Geometry check sheet. Reference: drawing and pictorial views, mm from the part's lowest x, y, z. A direction names the side the tool comes from. Give positions to 0.01 mm unless a question says otherwise; leave off trailing zeros. Order: outer loops, then holes, each group sorted by start corner. A loop starts at its lowest first (then second) coordinate and runs counter-clockwise, first axis right, second up. Notation, with made-up numbers: M 80,2 L 122,2 A29 cw 122,34 Z; hole C 16.25,19 d5. An arc over 180 degrees is marked long. Use CSV: the item, a comma, the result in double quotes. Start each with the question number.
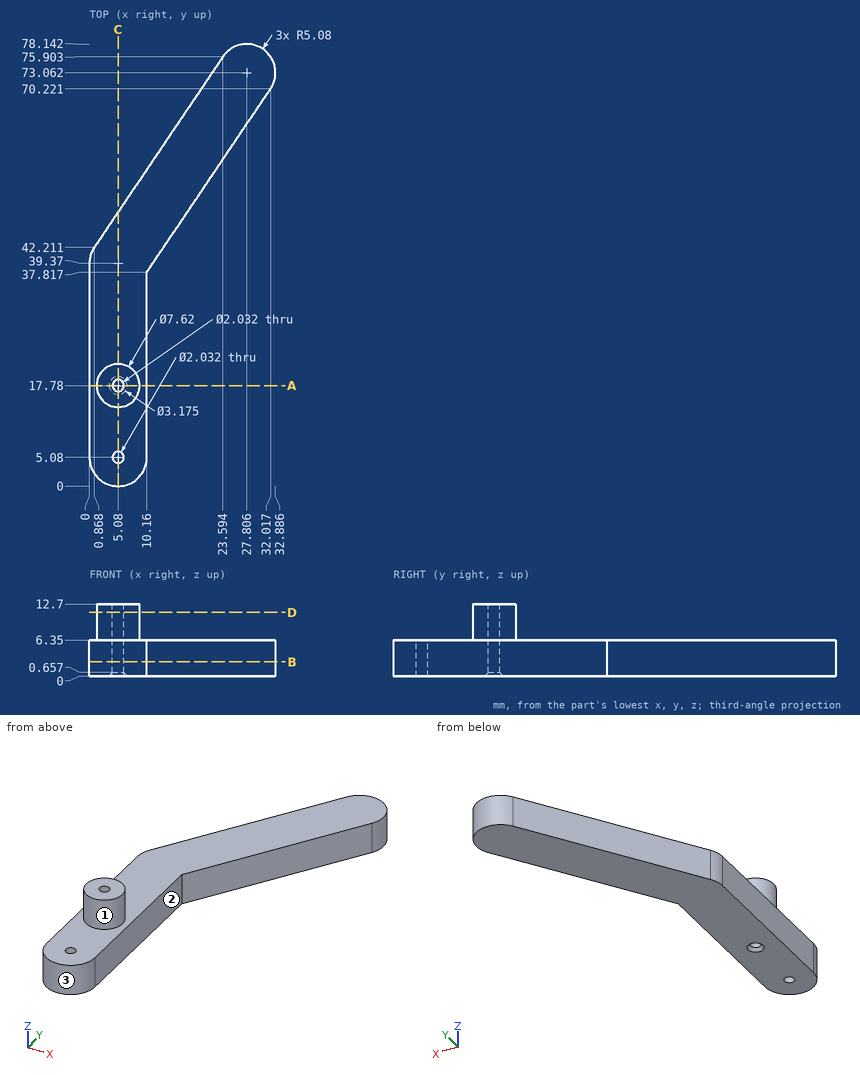
(1) Thickness scan on line 1 (Y direction, x = 5.08, z = 2.5) (1 decimal); line 2 (X direction, y = 17.78, z = 6) (1 decimal); line 3 (X direction, y = 31, z = 3.75). Record the ranges inside material, lowest first.
(2) Access from +Z, -Z, +X, -X, +Y, -Y to the whole of each face (thin tool, end or side, straight path). Record for the marked faces 1, 2 and 3.
(3) Sectioned sample at D-D on z = 11.25. Record the cut outline in (x, y).
(4) Go/stop test with flat-tipped pins: P1, Ø2, axis at x = 19.5, z = 9, coming from the -Y side; P2, Ø10, axis at x = 16.5, y = 65.5, coming from the +Z side; P3, Ø3, axis at y = 24.5, z = 2.5, coming from the +X side. Record where each tip stops, or that it passes through.
(5) Sectioned sample at A-A on y = 17.78. Record the cut outline in (x, z).
(6) Sectioned sample at C-C on x = 5.08. Give the number of separate pieces and of enclosed holes in the cut face, then the cut area to 3 significant figures.
(7) Sectioned sample at B-B on z = 2.5. Record the cut outline in (x, y) (1 decimal).
Responses:
1,line 1,"0 to 4.1, 6.1 to 16.8, 18.8 to 48.5"
1,line 2,"0 to 4.1, 6.1 to 10.2"
1,line 3,"0 to 10.16"
2,face 1,"+Z"
2,face 2,"+Z, -Z, +X, -Y"
2,face 3,"+Z, -Z, -Y"
3,outline,"C 5.08,17.78 d7.62; hole C 5.08,17.78 d2.03"
4,P1,"through"
4,P2,"z = 6.35"
4,P3,"x = 10.16"
5,outline,"M 0,0 L 3.49,0 L 4.06,0.66 L 4.06,12.7 L 1.27,12.7 L 1.27,6.35 L 0,6.35 Z; M 6.1,0.66 L 6.67,0 L 10.16,0 L 10.16,6.35 L 8.89,6.35 L 8.89,12.7 L 6.1,12.7 Z"
6,separate pieces,"3"
6,enclosed holes,"0"
6,area,"317 mm2"
7,outline,"M 0,5.1 A5.1 ccw 10.2,5.1 L 10.2,37.8 L 32,70.2 A5.1 ccw 23.6,75.9 L 0.9,42.2 A5.1 ccw 0,39.4 Z; hole C 5.1,5.1 d2; hole C 5.1,17.8 d2"
